Autodesk Inventor part; units mm, degrees
ref_plane "YZ Plane" through (0, 0, 0) normal (1, 0, 0) x (0, 1, 0)
ref_plane "XZ Plane" through (0, 0, 0) normal (0, 1, 0) x (-1, 0, 0)
ref_plane "XY Plane" through (0, 0, 0) normal (0, 0, 1) x (1, 0, 0)
sketch "Sketch_1" plane through (0, 0, 0) normal (0, 0, 1) x (1, 0, 0)
  line L0 (0, -3) -> (0, 14.5)
  line L1 (0, 14.5) -> (3.35, 14.5)
  line L2 (3.35, 14.5) -> (3.35, 13)
  line L3 (3.35, 13) -> (1.975, 13)
  line L4 (1.975, 13) -> (1.975, 12.1)
  line L5 (1.975, 12.1) -> (3.5, 12.1)
  line L6 (3.5, 12.1) -> (3.5, 0)
  line L7 (3.5, 0) -> (2.0095, 0)
  line L8 (2.0095, 0) -> (2.5, -0.4905)
  line L9 (2.5, -0.4905) -> (2.5, -2.5095)
  line L10 (2.5, -2.5095) -> (2.0095, -3)
  line L11 (2.0095, -3) -> (0, -3)
  line L12 (0, -3) -> (0, 14.5)
revolve "Revolution1" add sketch "Sketch_1" angle 360 about axis through (0, -3, 0) along (0, -1, 0)
thread "Thread1"
sketch "Sketch_2" plane through (0, 0, 0) normal (0, 0, 1) x (1, 0, 0)
  line L0 (0, 1.2) -> (0, 14.5)
  line L1 (0, 14.5) -> (1.6, 14.5)
  line L2 (1.6, 14.5) -> (1.6, 1.2)
  line L3 (1.6, 1.2) -> (0, 1.2)
  line L4 (0, 1.2) -> (0, 14.5)
revolve "Revolution2" cut sketch "Sketch_2" angle 360 about axis through (0, 1.2, 0) along (0, -1, 0)
sketch "Sketch_3" plane through (0, 14.5, 0) normal (0, 1, 0) x (1, 0, 0)
  line L0 (-1, 0.5774) -> (-1, -0.5774)
  line L1 (-1, -0.5774) -> (0, -1.1547)
  line L2 (0, -1.1547) -> (1, -0.5774)
  line L3 (1, -0.5774) -> (1, 0.5774)
  line L4 (1, 0.5774) -> (0, 1.1547)
  line L5 (0, 1.1547) -> (-1, 0.5774)
extrude "Extrusion1" cut sketch "Sketch_3" against normal blind 16.3
properties part number "KQ2S23-M5N N"
Here's how the part is built. I have some questions about the finished solid (model axes, mm). A direction names the side the tool comes from. Round coordinates to 2 decimals unless told otherwise and drop trailing zeros. Write each loop counter-clockwise with the first axis right and the second up, starting at its lowest first coordinate (ties: lowest second). Pieces come first, ordered by that corner, then holes.
1. I need wall thicknesses on L1, parallel to Y at x = -0.5, z = 2.75; L2, parallel to Y at x = 1.25, z = 2; L3, parallel to Z at x = 0, y = 11. Which ranges of each line are inside material? Lowest first, please.
2. For faces 1 (the flat face through (1, 0, 0)), 2 (the flat face through (2, 12.1, -2)), 3 (the flat face through (0, -3, 0)), 4 (the cylindrical face through (-0.54, -1.51, -2.44)), which set-ups out of +Z, -Z, +X, -X, +Y, -Y let a thin tool reach every point of the face, with its end or its side?
3. Suppose I cut it at D-D (y = 13.5). List the corners of the cut face in (x, z) for me, and give its area (3 significant figures).
4. If we mould it in two halves opening along Z, with no side actions, what happens to faces 5 (the cylindrical face through (-3.347, 13.74, 0.147)), 6 (the flat face through (-2, 14.5, -1)), 7 (the flat face through (-0.51, -0.28, 0.86))? For each: released by +Z, released by -Z, zero draft, split by the parting line, or undercut.
5. Suppose I cut it at A-A (y = -1). List the corners of the cut face in (x, z) for me, and give its area (3 significant figures).
6. Suppose I cut it at B-B (z = 3). List the corners of the cut face in (x, y) for me.
7. Will these pins go through, and if not, where does the flat tip stop? pin 1 Ø2.5 at (x, z) = (0, 0) entering from +Y; pin 2 Ø1 at (y, z) = (12, 1.5) entering from -X; pin 3 Ø2 at (y, z) = (4.5, 2) entering from +X.
Answer sheet:
1. L1: y = 0 to 12.1, 13 to 14.5
1. L2: y = -2.65 to -0.35, 0 to 12.1, 13 to 14.5
1. L3: z = -3.5 to -1.6, 1.6 to 3.5
2. face 1: +Y
2. face 2: none
2. face 3: +Z, -Z, +X, -X, -Y
2. face 4: -Y
3. outline: circle Ø6.7 at (0, 0); hole circle Ø3.2 at (0, 0)
3. area: 27.2 mm2
4. face 5: split by the parting line
4. face 6: zero draft
4. face 7: undercut
5. outline: circle Ø5 at (0, 0); hole (-1, -0.58) - (0, -1.15) - (1, -0.58) - (1, 0.58) - (0, 1.15) - (-1, 0.58) - close
5. area: 16.2 mm2
6. outline: (-1.8, 0) - (1.8, 0) - (1.8, 12.1) - (-1.8, 12.1) - close; (-1.49, 13) - (1.49, 13) - (1.49, 14.5) - (-1.49, 14.5) - close
7. pin 1: stops at y = 1.2
7. pin 2: stops at x = -3.35
7. pin 3: stops at x = 3.35
